```python
from build123d import *

# Parameters (mm, degrees)
F0_W     = 100
F0_H     = 100
F0_W_2   = 400
F1_DEPTH = 25
F3_DEPTH = 400
F4_R     = 15.5
F6_DEPTH = 40
F5_R     = 15.5
F7_DEPTH = 40


with BuildPart() as f1:
    # F0 (on Front) → F1 (new body, symmetric)
    with BuildSketch(Plane.XZ):
        Polygon((900, 200), (0, 200), (0, 150), (100, 150), (100, -200), (0, -200), (0, -250), (150, -250), (450, 0), (900, 0), align=None)
        Polygon((150, -184.914586), (150, 0), (371.897503, 0), align=None, mode=Mode.SUBTRACT)
        with Locations((200, 100)):
            Rectangle(F0_W, F0_H, mode=Mode.SUBTRACT)
        with Locations((350, 100)):
            Rectangle(F0_W, F0_H, mode=Mode.SUBTRACT)
        with Locations((650, 100)):
            Rectangle(F0_W_2, F0_H, mode=Mode.SUBTRACT)
    extrude(amount=F1_DEPTH, both=True)

    # F2 (on face) → F3 (join)
    with BuildSketch(Plane.YZ.offset(900)):
        Polygon((0, 217.67767), (-17.67767, 200), (17.67767, 200), align=None)
        Polygon((17.67767, 0), (-17.67767, 0), (0, -17.67767), align=None)
    extrude(amount=-F3_DEPTH)

    # F4 (on face) → F6 (join)
    with BuildSketch(Plane(origin=(0, 0, -250), x_dir=(1, 0, 0), z_dir=(0, 0, -1))):
        with Locations((30, 0)):
            Circle(F4_R)
    extrude(amount=F6_DEPTH)

    # F5 (on face) → F7 (join)
    with BuildSketch(Plane(origin=(0, 0, 150), x_dir=(1, 0, 0), z_dir=(0, 0, -1))):
        with Locations((30, 0)):
            Circle(F5_R)
    extrude(amount=F7_DEPTH)


solid = f1.part
```
Can you work these out from the model? Positions are in its coordinate system, mm. A direction names the side the tool comes from. Round coordinates to 2 decimals unless told otherwise and drop trailing zeros. Loops run counter-clockwise (first coordinate to the right, second up) from the corner with the lowest first, then second, coordinate; pieces in that order, holes last. Notation, with made-up numbers: (53, 69.5) -> (86, 69.5) arc R17 ccw to (86, 73.5) -> close; hole circle Ø7 at (38, 51). An arc over 180 degrees is marked (long way). One line per item, written item: value. Start each with the question number.
1. If we mould it in two halves opening along X, with no side actions, what happens to faces 4 (the flat face through (30, 0, -290)), 5 (the flat face through (500, 0, -7)), 6 (the flat face through (0, 0, 175))? For each: pulls with the +X half, pulls with the -X half, needs draft (parallel to the pull), parting line crosses it, or undercut.
2. If we section it at B-B, the plane x = 599: Write out the boundary of the cut face in (y, z).
3. For faces 1 (the flat face through (150, 0, 99)), 2 (the cylindrical face through (44.318, 5.937, 130.28)), 3 (the flat face through (30, 0, 110)), which set-ups out of +Z, -Z, +X, -X, +Y, -Y let a thin tool reach every point of the face, with its end or its side?
4. If we section it at A-A, the plane z = 132: Write out the boundary of the cut face in (x, y), then the cut area to 3 significant figures.
5. If we section it at C-C, the plane z = 72.5: Write out the boundary of the cut face in (x, y), then the cut area to 3 significant figures.
6. If I drill on probe 1 along X at (y, z) = (22, 121); probe 2 along Z at (x, y) = (658.5, -21); probe 3 along X at (y, z) = (0.5, -262), over which ranges is the centre line in solid material (lowest first)?
7. If we section it at D-D, the plane z = -135: Write out the boundary of the cut face in (x, y).
8. For pin 1 (25 mm diameter, centred on y = 0.5, z = 118, fed in from -X); pin 2 (15 mm diameter, centred on x = 205, y = 0, fed in from -Z); pin 3 (8 mm diameter, centred on y = -16, z = 125, fed in from -X), each with a flat end and sliding along its axis, tell me the tip position at first contact or that it passes through.
Calculated:
1. face 4: needs draft
1. face 5: undercut
1. face 6: pulls with the -X half
2. outline: (-25, 0) -> (-17.68, 0) -> (0, -17.68) -> (17.68, 0) -> (25, 0) -> (25, 50) -> (-25, 50) -> close; (-25, 150) -> (25, 150) -> (25, 200) -> (17.68, 200) -> (0, 217.68) -> (-17.68, 200) -> (-25, 200) -> close
3. face 1: +Y, -Y
3. face 2: none
3. face 3: -X, +Y, -Y
4. outline: circle Ø31 at (30, 0); (100, -25) -> (150, -25) -> (150, 25) -> (100, 25) -> close; (250, -25) -> (300, -25) -> (300, 25) -> (250, 25) -> close; (400, -25) -> (450, -25) -> (450, 25) -> (400, 25) -> close; (850, -25) -> (900, -25) -> (900, 25) -> (850, 25) -> close
4. area: 10,800 mm²
5. outline: (100, -25) -> (150, -25) -> (150, 25) -> (100, 25) -> close; (250, -25) -> (300, -25) -> (300, 25) -> (250, 25) -> close; (400, -25) -> (450, -25) -> (450, 25) -> (400, 25) -> close; (850, -25) -> (900, -25) -> (900, 25) -> (850, 25) -> close
5. area: 10,000 mm²
6. probe 1: x = 100 to 150, 250 to 300, 400 to 450, 850 to 900
6. probe 2: z = 0 to 50, 150 to 200
6. probe 3: x = 14.51 to 45.49
7. outline: (100, -25) -> (150, -25) -> (150, 25) -> (100, 25) -> close; (209.9, -25) -> (288, -25) -> (288, 25) -> (209.9, 25) -> close
8. pin 1: stops at x = 14.5
8. pin 2: stops at z = -210.42
8. pin 3: stops at x = 20.19
